Part model, mm, in its own coordinate system. A direction names the side the tool comes from. Give positions to 0.01 mm unless a question says otherwise; leave off trailing zeros. Order: outer loops, then holes, each group sorted by start corner. A loop starts at its lowest first (then second) coordinate and runs counter-clockwise, first axis right, second up.
1. Slice it at D-D on x = -12.5. Give the number of separate pieces and of enclosed holes in the cut face, and give its area (3 significant figures).
2. Slice it at A-A on z = 0. List the corners of the cut face in (x, y), and give its area (3 significant figures).
3. Drop flat-ended pins along their axis: pin 1 Ø7 at (y, z) = (23, 1) entering from -X; pin 2 Ø2 at (x, y) = (3.5, 35.5) entering from -Z; pin 3 Ø6.5 at (x, z) = (-12.5, -15) entering from -Y; pin 4 Ø5 at (x, z) = (13.5, -8) entering from +Y. Give the stop position or say it passes through.
4. Probe line 1 (X direction, y = 3, z = -15); line 2 (Y direction, x = -0.5, z = 0); line 3 (Z direction, x = -12, y = 5). List the from-to ranges inside material, lowest first.
5. Mould opens along Z. For faces 1 (the flat face through (-7.5, 18, -4)), 2 (the flat face through (0, 11, 20)), 3 (the cylindrical face through (-10.517, 4.192, 14.74)) say: +Z half, -Z half, draft (parallel to the pull), parting line (faces both ways), or undercut.
6. Slice it at C-C on y = 25. List the corners of the cut face in (x, z).
7. Slice it at B-B on x = 1.5. List the corners of the cut face in (y, z).
8. Which spindle directions (+Z, -Z, +X, -X, +Y, -Y) get a long thin tool onto all of the face, cutting with end or side? Do faces 4 (the cylindrical face through (14.483, 4.192, -15.26)), 5 (the flat face through (7.5, 25.2, -4.2)), 6 (the cylindrical face through (-4.965, 18.166, 1.517)). Say none if no direction does.
from build123d import *
from OCP.BRepFilletAPI import BRepFilletAPI_MakeChamfer

# Parameters (mm, degrees)
SKETCH_2_W          = 35
SKETCH_2_H          = 40
EXTRUDE_1_DEPTH     = 10
SKETCH_3_R          = 2
CUT_EXTRUDE_2_DEPTH = 10
SKETCH_4_W          = 15
SKETCH_4_H          = 40
EXTRUDE_2_DEPTH     = 30
SKETCH_5_R          = 7
CUT_EXTRUDE_3_DEPTH = 52.23475383
FILLET_2_R          = 3
FILLET_3_R          = 10
CHAMFER_1_SIZE      = 3
CHAMFER_1_SIZE_2    = 1.732050808
SKETCH_6_R          = 7
SKETCH_6_R_2        = 4.05
EXTRUDE_3_DEPTH     = 10


with BuildPart() as part:
    # 草图2 → 凸台-拉伸1 (new body)
    with BuildSketch(Plane(origin=(0, 0, 0), x_dir=(1, 0, 0), z_dir=(0, 1, 0))):
        Rectangle(SKETCH_2_W, SKETCH_2_H)
    extrude(amount=EXTRUDE_1_DEPTH)

    # 草图3 → 切除-拉伸2 (cut)
    with BuildSketch(Plane(origin=(0, 10, 0), x_dir=(1, 0, 0), z_dir=(0, 1, 0))):
        with Locations(Location((12.5, 15, 0), (0, 0, 270))):
            Circle(SKETCH_3_R)
        with Locations(Location((-12.5, 15, 0), (0, 0, 270))):
            Circle(SKETCH_3_R)
        with Locations(Location((-12.5, -15, 0), (0, 0, 270))):
            Circle(SKETCH_3_R)
        with Locations(Location((12.5, -15, 0), (0, 0, 270))):
            Circle(SKETCH_3_R)
    extrude(amount=-CUT_EXTRUDE_2_DEPTH, mode=Mode.SUBTRACT)

    # 草图4 → 凸台-拉伸2 (add)
    with BuildSketch(Plane(origin=(0, 10, 0), x_dir=(1, 0, 0), z_dir=(0, 1, 0))):
        Rectangle(SKETCH_4_W, SKETCH_4_H)
    extrude(amount=EXTRUDE_2_DEPTH)

    # 草图5 → 切除-拉伸3 (cut, through all)
    with BuildSketch(Plane(origin=(7.5, 0, 0), x_dir=(0, 0, -1), z_dir=(1, 0, 0))):
        with Locations((0, 25)):
            Circle(SKETCH_5_R)
    extrude(amount=-CUT_EXTRUDE_3_DEPTH, mode=Mode.SUBTRACT)

    # 圆角2
    fillet_2_edges = [part.edges().sort_by_distance(p)[0] for p in [
        (17.5, 5, -20),
        (-17.5, 5, -20),
        (-17.5, 5, 20),
        (17.5, 5, 20),
    ]]
    fillet(fillet_2_edges, radius=FILLET_2_R)

    # 圆角3
    fillet_3_edges = [part.edges().sort_by_distance(p)[0] for p in [
        (0, 40, 20),
        (0, 40, -20),
    ]]
    fillet(fillet_3_edges, radius=FILLET_3_R)

    # 倒角1
    chamfer_1_edges_1 = [part.edges().sort_by_distance(p)[0] for p in [
        (-12.5, 10, -17),
    ]]
    chamfer_1_side_1 = [part.faces().sort_by_distance(p)[0] for p in [
        (-12.5, 10, -17.034641016),
    ]]
    chamfer_1_edges_2 = [part.edges().sort_by_distance(p)[0] for p in [
        (-12.5, 10, 13),
    ]]
    chamfer_1_side_2 = [part.faces().sort_by_distance(p)[0] for p in [
        (-12.5, 10, 12.965358984),
    ]]
    chamfer_1_edges_3 = [part.edges().sort_by_distance(p)[0] for p in [
        (12.5, 10, 13),
    ]]
    chamfer_1_side_3 = [part.faces().sort_by_distance(p)[0] for p in [
        (12.5, 10, 12.965358984),
    ]]
    chamfer_1_edges_4 = [part.edges().sort_by_distance(p)[0] for p in [
        (12.5, 10, -17),
    ]]
    chamfer_1_side_4 = [part.faces().sort_by_distance(p)[0] for p in [
        (12.5, 10, -17.034641016),
    ]]
    chamfer_1 = BRepFilletAPI_MakeChamfer(part.part.solid().wrapped)
    for e in chamfer_1_edges_1:
        chamfer_1.Add(CHAMFER_1_SIZE - 0.0001, CHAMFER_1_SIZE_2 - 0.0001, e.wrapped, chamfer_1_side_1[0].wrapped)
    for e in chamfer_1_edges_2:
        chamfer_1.Add(CHAMFER_1_SIZE - 0.0001, CHAMFER_1_SIZE_2 - 0.0001, e.wrapped, chamfer_1_side_2[0].wrapped)
    for e in chamfer_1_edges_3:
        chamfer_1.Add(CHAMFER_1_SIZE - 0.0001, CHAMFER_1_SIZE_2 - 0.0001, e.wrapped, chamfer_1_side_3[0].wrapped)
    for e in chamfer_1_edges_4:
        chamfer_1.Add(CHAMFER_1_SIZE - 0.0001, CHAMFER_1_SIZE_2 - 0.0001, e.wrapped, chamfer_1_side_4[0].wrapped)
    add(Compound.cast(chamfer_1.Shape()), mode=Mode.REPLACE)  # a hair under: the kernel refuses the full size

    # 草图6 → 凸台-拉伸3 (add)
    with BuildSketch(Plane(origin=(7.5, 0, 0), x_dir=(0, 0, -1), z_dir=(1, 0, 0))):
        with Locations((0, 25)):
            Circle(SKETCH_6_R)
        with Locations((0, 25)):
            Circle(SKETCH_6_R_2, mode=Mode.SUBTRACT)
    extrude(amount=-EXTRUDE_3_DEPTH)


solid = part.part
Data:
1. separate pieces: 3
1. enclosed holes: 0
1. area: 310 mm2
2. outline: (-17.5, 0) - (17.5, 0) - (17.5, 10) - (7.5, 10) - (7.5, 20.95) - (-2.5, 20.95) - (-2.5, 18) - (-7.5, 18) - (-7.5, 10) - (-17.5, 10) - close; (-7.5, 32) - (-2.5, 32) - (-2.5, 29.05) - (7.5, 29.05) - (7.5, 40) - (-7.5, 40) - close
2. area: 649 mm2
3. pin 1: stops at x = -2.5
3. pin 2: stops at z = -18.93
3. pin 3: stops at y = 0
3. pin 4: stops at y = 10
4. line 1: x = -17.5 to -14.5, -10.5 to 10.5, 14.5 to 17.5
4. line 2: y = 0 to 20.95, 29.05 to 40
4. line 3: z = -20 to -16.94, -13.06 to 13.06, 16.94 to 20
5. face 1: draft
5. face 2: +Z half
5. face 3: undercut
6. outline: (-7.5, -20) - (7.5, -20) - (7.5, -4.05) - (-2.5, -4.05) - (-2.5, -7) - (-7.5, -7) - close; (-7.5, 7) - (-2.5, 7) - (-2.5, 4.05) - (7.5, 4.05) - (7.5, 20) - (-7.5, 20) - close
7. outline: (0, -20) - (30, -20) arc R10 ccw to (40, -10) - (40, 10) arc R10 ccw to (30, 20) - (0, 20) - close; hole circle Ø8.1 at (25, 0)
8. face 4: +Y, -Y
8. face 5: +Z, -Z, +X, +Y
8. face 6: -X
